Read the model definition and answer for the solid it produces. Units are mm, in the model's axes. Face numbers are marked on the shaded views. A direction names the side the tool comes from. Coordinates: 2 decimals unless noted, no trailing zeros. Write each loop counter-clockwise with the first axis right and the second up, starting at its lowest first coordinate (ties: lowest second). Pieces come first, ordered by that corner, then holes.
(1) Straight lines are drawn through the part: line 1 along Z through (x, y) = (-3.6, 0); line 2 along X through (y, z) = (3.35, 0); line 3 along Y through (x, z) = (-0.5, -2.25). For each, find the intervals that lie inside material, in ascending order.
(2) The part is cut by section A-A, the plane y = -3. Determine the outline of the cut face in (x, z).
(3) The part is cut by section B-B, the plane x = -0.25. Determine the outline of the cut face in (y, z).
(4) The part is cut by section D-D, the plane z = -4. Determine the outline of the cut face in (x, y).
(5) The part is cut by section C-C, the plane z = 0. Determine the outline of the cut face in (x, y), and give its area (3 significant figures).
(6) Which of the six approach directions +Z, -Z, +X, -X, +Y, -Y give full straight-line access (tool end or side, diameter ignored) to the marked faces 1, 2 and 3?
(7) Determine the mould class of the marked faces 4, 5 and 6 for opening direction Y: pulls with the +Y half, pulls with the -Y half, needs draft (parallel to the pull), parting line crosses it, or undercut.
(8) Given pin 1 (1.5 mm diameter, centred on x = -3, z = 2.5, fed in from -Y); pin 2 (3 mm diameter, centred on x = 1, y = -2.5, fed in from +Z); pin 3 (1.6 mm diameter, centred on y = 0, z = 0, fed in from -X); pin 4 (2 mm diameter, centred on x = 1.59, z = 0, fed in from +Y), each flat-ended and moving along its own axis, determine where each tip first touches the part or whether it passes through.
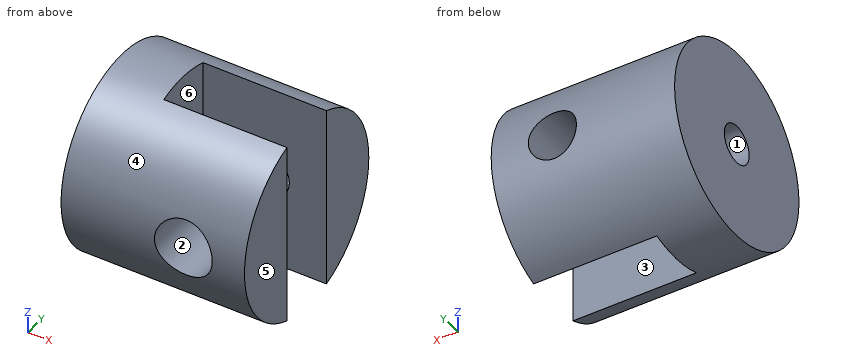
```python
from build123d import *

# Parameters (mm, degrees)
F0_R     = 5
F1_DEPTH = 4.7625
F3_D     = 1.9939
F3_DEPTH = 2.9416666667
F3_TIP   = 0.5990279941
F4_W     = 12.8
F4_H     = 3.175
F5_DEPTH = 12.5
F7_D     = 2.5
F7_DEPTH = 3.4135
F8_R     = 1.5
F9_DEPTH = 3.4135001


with BuildPart() as f1:
    # F0 (on Right) → F1 (new body, symmetric)
    with BuildSketch(Plane.YZ):
        Circle(F0_R)
    extrude(amount=F1_DEPTH, both=True)

    # F3
    with Locations(Plane(origin=(-4.7625, 0, 0), x_dir=(0, -1, 0), z_dir=(-1, 0, 0))):
        with Locations((0, 0)):
            Hole(F3_D / 2, depth=F3_DEPTH)
            with Locations((0, 0, -(F3_DEPTH + F3_TIP / 2))):  # 118° drill point
                Cone(0, F3_D / 2, F3_TIP, mode=Mode.SUBTRACT)

    # F4 (on Top) → F5 (cut, symmetric)
    with BuildSketch(Plane.XY):
        with Locations((4.7625, 0)):
            Rectangle(F4_W, F4_H)
    extrude(amount=F5_DEPTH, both=True, mode=Mode.SUBTRACT)

    # F7 (through all, one way)
    with BuildSketch(Plane.XZ.offset(-1.5875)):
        with Locations((1.5875, 0)):
            Circle(F7_D / 2)
    extrude(amount=-F7_DEPTH, mode=Mode.SUBTRACT)

    # F8 (on face) → F9 (cut, through all)
    with BuildSketch(Plane(origin=(0, -1.5875, 0), x_dir=(-1, 0, 0), z_dir=(0, 1, 0))):
        with Locations((-1.5875, 0)):
            Circle(F8_R)
    extrude(amount=-F9_DEPTH, mode=Mode.SUBTRACT)


solid = f1.part
```
Computed:
1. line 1: z = -5 to -1, 1 to 5
1. line 2: x = -4.76 to 0.34, 2.84 to 4.76
1. line 3: y = -4.47 to -1.59, 1.59 to 4.47
2. outline: (-4.76, -4) - (4.76, -4) - (4.76, 4) - (-4.76, 4) - close; hole circle Ø3 at (1.59, 0)
3. outline: (-1.59, -4.74) - (-1.59, 4.74) arc R5 ccw to start; (1.59, -4.74) arc R5 ccw to (1.59, 4.74) - close
4. outline: (-4.76, -3) - (4.76, -3) - (4.76, -1.59) - (-1.64, -1.59) - (-1.64, 1.59) - (4.76, 1.59) - (4.76, 3) - (-4.76, 3) - close
5. outline: (-4.76, -5) - (0.09, -5) - (0.09, -1.59) - (-1.64, -1.59) - (-1.64, -0.69) - (-1.82, -1) - (-4.76, -1) - close; (-4.76, 1) - (-1.82, 1) - (-1.64, 0.69) - (-1.64, 1.59) - (0.34, 1.59) - (0.34, 5) - (-4.76, 5) - close; (2.84, 1.59) - (4.76, 1.59) - (4.76, 5) - (2.84, 5) - close; (3.09, -5) - (4.76, -5) - (4.76, -1.59) - (3.09, -1.59) - close
5. area: 50.0 mm2
6. face 1: -X
6. face 2: -Y
6. face 3: +Z, -Z, +X
7. face 4: parting line crosses it
7. face 5: needs draft
7. face 6: undercut
8. pin 1: stops at y = -4.68
8. pin 2: stops at z = 4.74
8. pin 3: stops at x = -1.7
8. pin 4: passes through
